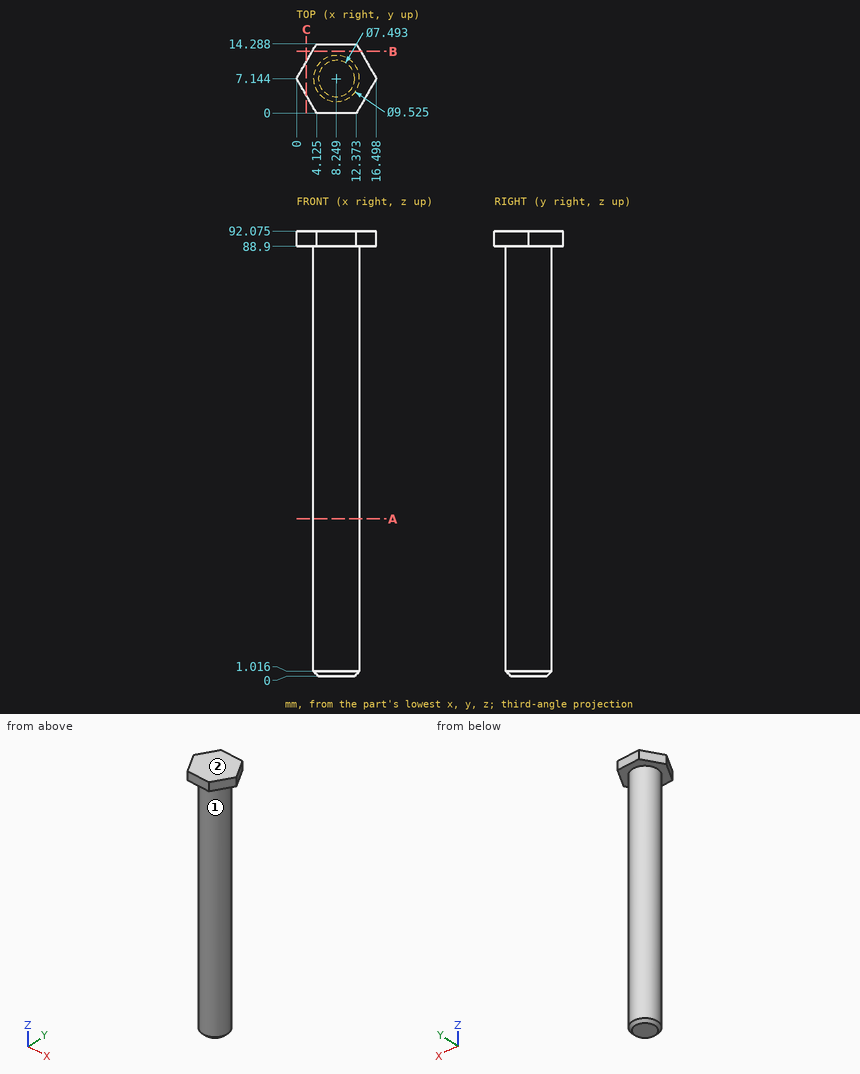
Answer from the drawing. Dimensions are ordinates in mm from the lowest x, y and z of the part. A direction names the side the tool comes from. Coordinates: 2 decimals unless noted, no trailing zeros. Loops run counter-clockwise (first coordinate to the right, second up) from the corner with the lowest first, then second, coordinate; pieces in that order, holes last.
Q1. The part is cut by section B-B on y = 12.75. Write down the section's boundary in (x, z) (1 decimal).
Q2. Which of the six approach directions +Z, -Z, +X, -X, +Y, -Y give full straight-line access (tool end or side, diameter ignored) to the marked faces 1 and 2?
Q3. Each of these flat-tipped pins is pushed along its axis until it touches: pin 1 Ø5 at (x, z) = (9.5, 69) entering from +Y; pin 2 Ø7 at (x, y) = (10.5, 5.5) entering from -Z; pin 3 Ø4 at (x, z) = (8, 69.5) entering from -Y; pin 4 Ø4 at (x, y) = (13, 3) entering from -Z. Where does it stop, or does it pass through?
Q4. The part is cut by section A-A on z = 32.5. Write down the section's boundary in (x, y) (1 decimal).
Q5. The part is cut by section C-C on x = 2. Write down the section's boundary in (y, z) (1 decimal).
Q6. Consider probe 1 along Y at (x, z) = (8.25, 46); probe 2 along X at (y, z) = (7.25, 61); probe 3 along Z at (x, y) = (3.5, 3) (1 decimal). Determine where each line is inside the solid, lowest interval first.
Results below:
1. outline: (3.2, 88.9) - (13.3, 88.9) - (13.3, 92.1) - (3.2, 92.1) - close
2. face 1: -Z
2. face 2: +Z, +X, -X, +Y, -Y
3. pin 1: stops at y = 11.91
3. pin 2: stops at z = 0
3. pin 3: stops at y = 2.38
3. pin 4: stops at z = 0.56
4. outline: circle Ø9.5 at (8.2, 7.1)
5. outline: (3.7, 88.9) - (10.6, 88.9) - (10.6, 92.1) - (3.7, 92.1) - close
6. probe 1: y = 2.38 to 11.91
6. probe 2: x = 3.49 to 13.01
6. probe 3: z = 88.9 to 92.1
